```python
from build123d import *

# Parameters (mm, degrees)
SKETCH_1_R          = 16
EXTRUDE_1_DEPTH     = 9
SKETCH_2_R          = 6
EXTRUDE_2_DEPTH     = 0.5
SKETCH_3_R          = 16
EXTRUDE_3_DEPTH     = 3.25
SKETCH_4_R          = 5.5
EXTRUDE_4_DEPTH     = 2.25
SKETCH_5_R          = 3
CUT_EXTRUDE_1_DEPTH = 26.25
SKETCH_6_R          = 8
SKETCH_6_R_2        = 5.5
CUT_EXTRUDE_2_DEPTH = 2.25
SKETCH_7_R          = 0.6
CUT_EXTRUDE_3_DEPTH = 6
SKETCH_8_R          = 0.6
CUT_EXTRUDE_4_DEPTH = 3
SKETCH_9_R          = 18.290801542
SKETCH_9_R_2        = 5.5
CUT_EXTRUDE_5_DEPTH = 3.75


with BuildPart() as part:
    # 草图1 → 凸台-拉伸1 (new body)
    with BuildSketch(Plane.XY):
        Circle(SKETCH_1_R)
    extrude(amount=EXTRUDE_1_DEPTH)

    # 草图2 → 凸台-拉伸2 (add)
    with BuildSketch(Plane.XY.offset(9)):
        Circle(SKETCH_2_R)
    extrude(amount=EXTRUDE_2_DEPTH)

    # 草图3 → 凸台-拉伸3 (add)
    with BuildSketch(Plane.XY.offset(9.5)):
        Circle(SKETCH_3_R)
    extrude(amount=EXTRUDE_3_DEPTH)

    # 草图4 → 凸台-拉伸4 (add)
    with BuildSketch(Plane.XY.offset(12.75)):
        Circle(SKETCH_4_R)
    extrude(amount=EXTRUDE_4_DEPTH)

    # 草图5 → 切除-拉伸1 (cut)
    with BuildSketch(Plane.XY.offset(15)):
        Circle(SKETCH_5_R)
    extrude(amount=-CUT_EXTRUDE_1_DEPTH, mode=Mode.SUBTRACT)

    # 草图6 → 切除-拉伸2 (cut)
    with BuildSketch(Plane.XY.offset(12.75)):
        Circle(SKETCH_6_R)
        Circle(SKETCH_6_R_2, mode=Mode.SUBTRACT)
    extrude(amount=-CUT_EXTRUDE_2_DEPTH, mode=Mode.SUBTRACT)

    # 草图7 → 切除-拉伸3 (cut)
    with BuildSketch(Plane(origin=(0, 0, 0), x_dir=(-1, 0, 0), z_dir=(0, 0, -1))):
        with Locations((8.660254038, 5)):
            Circle(SKETCH_7_R)
        with Locations((-8.660254038, 5)):
            Circle(SKETCH_7_R)
        with Locations((0, -10)):
            Circle(SKETCH_7_R)
    extrude(amount=-CUT_EXTRUDE_3_DEPTH, mode=Mode.SUBTRACT)

    # 草图8 → 切除-拉伸4 (cut)
    with BuildSketch(Plane.XY.offset(12.75)):
        with Locations((5, -8.660254038)):
            Circle(SKETCH_8_R)
        with Locations((5, 8.660254038)):
            Circle(SKETCH_8_R)
        with Locations((-10, 0)):
            Circle(SKETCH_8_R)
    extrude(amount=-CUT_EXTRUDE_4_DEPTH, mode=Mode.SUBTRACT)

    # 草图9 → 切除-拉伸5 (cut)
    with BuildSketch(Plane.XY.offset(12.75)):
        Circle(SKETCH_9_R)
        Circle(SKETCH_9_R_2, mode=Mode.SUBTRACT)
    extrude(amount=-CUT_EXTRUDE_5_DEPTH, mode=Mode.SUBTRACT)


solid = part.part
```
Part model, mm, in its own coordinate system. A direction names the side the tool comes from. Coordinates: 2 decimals unless noted, no trailing zeros. Loops run counter-clockwise (first coordinate to the right, second up) from the corner with the lowest first, then second, coordinate; pieces in that order, holes last. Notation, with made-up numbers: (-1, 22.25) - (22, 22.25) arc R15 ccw to (22, 47.25) - close; hole circle Ø5 at (22, -28). An arc over 180 degrees is marked (long way). Write item = value, one per line. Start each with the question number.
Item 1: Cut at D-D, the plane y = 5. Give the cut face in (x, z), and give its area (3 significant figures).
Item 2: Cut at C-C, the plane z = 3.5. Give the cut face in (x, y), and give its area (3 significant figures).
Item 3: Flat gauge pins, fed straight in: pin 1 Ø5 at (x, z) = (7.5, 13.5) entering from -Y; pin 2 Ø8 at (y, z) = (-3, 13.5) entering from -X; pin 3 Ø1 at (x, y) = (0, -10) entering from -Z. Where does each tip first touch, or does it go through?
Item 4: 3-axis set-ups, long thin cutter, end or side, ignore diameter. For faces 4 (the cylindrical face through (-9.215, 4.77, 2.958)), 5 (the flat face through (7, 0, 9)), 6 (the cylindrical face through (-3, 0, 8)): which of +Z, -Z, +X, -X, +Y, -Y reach the whole face in a straight line?
Item 5: Cut at B-B, the plane x = 0. Give the cut face in (y, z).
Item 6: Mould opens along Y. For faces 1 (the flat face through (3.3, 0.2, 0)), 2 (the cylindrical face through (-1.19, -5.37, 12.04)), 3 (the flat face through (9, 5, 6)) say: released by +Y, released by -Y, zero draft, split by the parting line, or undercut.
Item 7: Wall check: L1, parallel to Y at x = 0, z = 4.45; L2, parallel to Z at x = 14, y = -1; L3, parallel to X at y = 1, z = 13.25. Give the ranges that are in metal, low to high. Write a range as from..to.
Item 8: Cut at A-A, the plane y = 0. Give the cut face in (x, z).
The answers:
q1.outline = (-15.2, 0) - (-9.26, 0) - (-9.26, 6) - (-8.06, 6) - (-8.06, 0) - (8.06, 0) - (8.06, 6) - (9.26, 6) - (9.26, 0) - (15.2, 0) - (15.2, 9) - (2.29, 9) - (2.29, 15) - (-2.29, 15) - (-2.29, 9) - (-15.2, 9) - close
q1.area = 287 mm2
q2.outline = circle Ø32 at (0, 0); hole circle Ø1.2 at (-8.66, 5); hole circle Ø6 at (0, 0); hole circle Ø1.2 at (0, -10); hole circle Ø1.2 at (8.66, 5)
q2.area = 773 mm2
q3.pin_1 = -2.29
q3.pin_2 = -5.5
q3.pin_3 = 6
q4.face_4 = -Z
q4.face_5 = +Z
q4.face_6 = +Z, -Z
q5.outline = (-16, 0) - (-10.6, 0) - (-10.6, 6) - (-9.4, 6) - (-9.4, 0) - (-3, 0) - (-3, 15) - (-5.5, 15) - (-5.5, 9) - (-16, 9) - close; (3, 0) - (16, 0) - (16, 9) - (5.5, 9) - (5.5, 15) - (3, 15) - close
q6.face_1 = zero draft
q6.face_2 = split by the parting line
q6.face_3 = undercut
q7.L1 = -16..-10.6, -9.4..-3, 3..16
q7.L2 = 0..9
q7.L3 = -5.41..-2.83, 2.83..5.41
q8.outline = (-16, 0) - (-3, 0) - (-3, 15) - (-5.5, 15) - (-5.5, 9) - (-16, 9) - close; (3, 0) - (16, 0) - (16, 9) - (5.5, 9) - (5.5, 15) - (3, 15) - close
